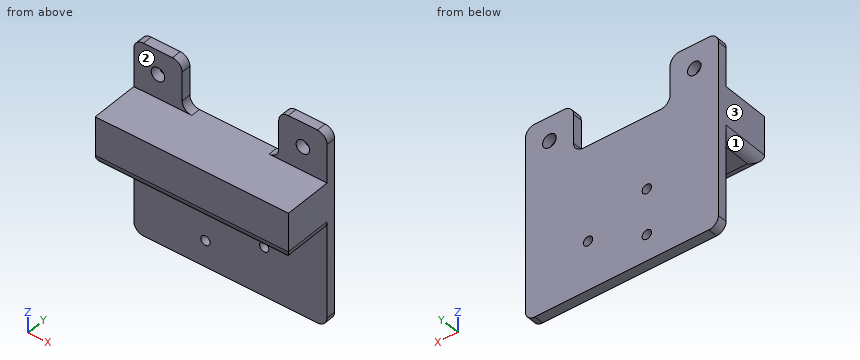
```python
from build123d import *

# Parameters (mm, degrees)
SKETCH_1_R      = 2.1
SKETCH_1_R_2    = 1.45
EXTRUDE_1_DEPTH = 3
SKETCH_2_W      = 60
SKETCH_2_H      = 15
EXTRUDE_2_DEPTH = 15
FILLET_1_R      = 3


with BuildPart() as part:
    # 草图1 → 凸台-拉伸1 (new body)
    with BuildSketch(Plane(origin=(0, 0, 0), x_dir=(1, 0, 0), z_dir=(0, 1, 0))):
        Polygon((-15, 7.5), (-15, -7.5), (-30, -7.5), (-30, 52.5), (30, 52.5), (30, -7.5), (15, -7.5), (15, 7.5), align=None)
        with Locations(Location((-22.5, 0, 0), (0, 0, 270))):
            Circle(SKETCH_1_R, mode=Mode.SUBTRACT)
        with Locations(Location((22.5, 0, 0), (0, 0, 90))):
            Circle(SKETCH_1_R, mode=Mode.SUBTRACT)
        with Locations(Location((-7.75, 44.3, 0), (0, 0, 270))):
            Circle(SKETCH_1_R_2, mode=Mode.SUBTRACT)
        with Locations(Location((10.5, 37.2, 0), (0, 0, 270))):
            Circle(SKETCH_1_R_2, mode=Mode.SUBTRACT)
        with Locations(Location((-7.75, 30.1, 0), (0, 0, 270))):
            Circle(SKETCH_1_R_2, mode=Mode.SUBTRACT)
    extrude(amount=EXTRUDE_1_DEPTH)

    # 草图2 → 凸台-拉伸2 (add)
    with BuildSketch(Plane.XZ):
        with Locations((0, -15)):
            Rectangle(SKETCH_2_W, SKETCH_2_H)
    extrude(amount=EXTRUDE_2_DEPTH)

    # 圆角1
    fillet_1_edges = [part.edges().sort_by_distance(p)[0] for p in [
        (-30, 1.5, -52.5),
        (30, 1.5, -52.5),
        (30, 1.5, 7.5),
        (15, 1.5, 7.5),
        (15, 1.5, -7.5),
        (-15, 1.5, -7.5),
        (-15, 1.5, 7.5),
        (-30, 1.5, 7.5),
        (-30, -7.5, -22.5),
        (30, -7.5, -22.5),
        (0, -15, -22.5),
    ]]
    fillet(fillet_1_edges, radius=FILLET_1_R)


solid = part.part
```
Could you check a few things on this model? Use its own coordinates, in mm. Face numbers are marked on the shaded views. A direction names the side the tool comes from. Give positions to 0.01 mm unless a question says otherwise; leave off trailing zeros. Write each loop counter-clockwise with the first axis right and the second up, starting at its lowest first coordinate (ties: lowest second). Pieces come first, ordered by that corner, then holes. Notation, with made-up numbers: (-3, 63.25) - (19, 63.25) arc R14 ccw to (19, 90.25) - close; hole circle Ø1 at (88.25, 73). An arc over 180 degrees is marked (long way). One line per item, written item: value. Start each with the question number.
Item 1: Please list where these lines run through material, in increasing order: line 1 (X direction, y = 2, z = -30.1); line 2 (Y direction, x = 27, z = 5.5); line 3 (Z direction, x = -1.5, y = -10.5). Write a range as from..to.
Item 2: Which directions (+Z, -Z, +X, -X, +Y, -Y) give clear straight access to the entire face, cutting with the end or side of a thin tool? Please do the marked faces 1, 2 and 3.
Item 3: Imagine slicing it at C-C, the plane z = 0. List the corners of the cut face in (x, y) for me.
Item 4: Imagine slicing it at B-B, the plane x = 10.5. List the corners of the cut face in (y, z) for me.
Item 5: Imagine slicing it at A-A, the plane x = -7.75. List the corners of the cut face in (y, z) for me, and give its area (3 significant figures).
Item 6: I'm going to push flat-ended pins straight in: pin 1 (5.5 mm diameter, centred on x = 22.5, z = 0, fed in from +Y); pin 2 (4.5 mm diameter, centred on x = -7.75, z = -30.1, fed in from -Y); pin 3 (4 mm diameter, centred on x = 5.5, y = -3.5, fed in from -Z). Where does each tip first touch, or does it pass through?
Item 7: Imagine slicing it at D-D, the plane z = -37.2. List the corners of the cut face in (x, y) for me.
Geometry says:
1. line 1: -30..-9.2, -6.3..30
1. line 2: 0..3
1. line 3: -22.5..-7.5
2. face 1: -Z, -X, -Y
2. face 2: +Z, +X, -X, -Y
2. face 3: +Z, -Z, -X, +Y, -Y
3. outline: (-30, 0) - (-24.6, 0) - (-24.6, 3) - (-30, 3) - close; (-20.4, 0) - (-15, 0) - (-15, 3) - (-20.4, 3) - close; (15, 0) - (20.4, 0) - (20.4, 3) - (15, 3) - close; (24.6, 0) - (30, 0) - (30, 3) - (24.6, 3) - close
4. outline: (-15, -19.5) arc R3 ccw to (-12, -22.5) - (0, -22.5) - (0, -35.75) - (3, -35.75) - (3, -7.5) - (-15, -7.5) - close; (0, -52.5) - (3, -52.5) - (3, -38.65) - (0, -38.65) - close
5. outline: (-15, -19.5) arc R3 ccw to (-12, -22.5) - (0, -22.5) - (0, -28.65) - (3, -28.65) - (3, -7.5) - (-15, -7.5) - close; (0, -52.5) - (3, -52.5) - (3, -45.75) - (0, -45.75) - close; (0, -42.85) - (3, -42.85) - (3, -31.55) - (0, -31.55) - close
5. area: 341 mm^2
6. pin 1: y = 3
6. pin 2: y = 0
6. pin 3: z = -22.5
7. outline: (-30, 0) - (9.05, 0) - (9.05, 3) - (-30, 3) - close; (11.95, 0) - (30, 0) - (30, 3) - (11.95, 3) - close
